CAD build for the part. Positions are in the model's coordinates, mm. Face numbers are marked on the shaded views. A direction names the side the tool comes from. Give positions to 0.01 mm unless a question says otherwise; leave off trailing zeros. Order: outer loops, then holes, each group sorted by start corner. A loop starts at its lowest first (then second) coordinate and runs counter-clockwise, first axis right, second up. Notation, with made-up numbers: (18, 16) -> (24, 16) arc R24 ccw to (24, 50) -> close; hole circle Ø1 at (17.5, 10.5). An arc over 180 degrees is marked (long way). Use one line per item in the form item = value. Start each with the question number.
1) Drop flat-ended pins along their axis: P1, Ø10, axis at y = 17.5, z = 31, coming from the +X side; P2, Ø3.5, axis at x = -60, y = 37, coming from the +Z side; P3, Ø0.9, axis at x = 60.5, y = -37, coming from the +Z side; P4, Ø1, axis at x = 59, z = 25.5, coming from the -Y side. Give the stop position or say it passes through.
2) Cut at A-A, the plane y = 0. State how many separate pieces and enclosed holes the cut face has, and give its area (3 significant figures).
3) Cut at B-B, the plane z = 23. Give the cut face in (x, y), and give its area (3 significant figures).
4) Mould opens along Y. For the marked faces 1, 2 and 3 say: pulls with the +Y half, pulls with the -Y half, needs draft (parallel to the pull), parting line crosses it, or undercut.
5) Tool access for the marked faces 4, 5, 6 and 7: list every direction of +Z, -Z, +X, -X, +Y, -Y with a clear straight run to the whole face (end or side of a thin tool).
6) Probe line 1 (Y direction, x = 60, z = 23); line 2 (Y direction, x = 45, z = 26); line 3 (X direction, y = 7.5, z = 14.5). List the from-to ranges inside material, lowest first.
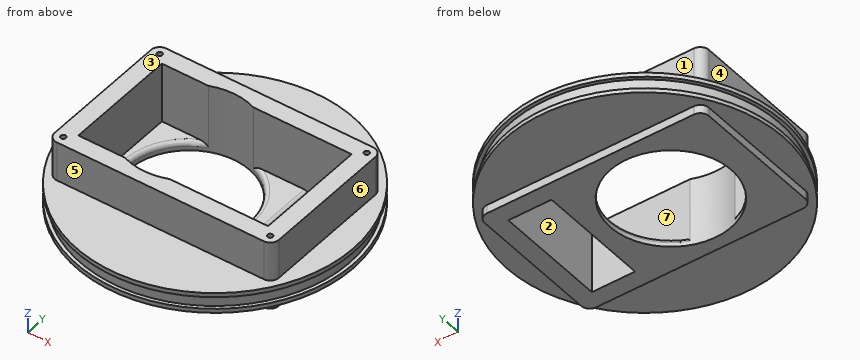
from build123d import *

# Parameters (mm, degrees)
SKETCH1_W           = 130
SKETCH1_H           = 85
SKETCH1_W_2         = 110
SKETCH1_H_2         = 65
BOSS_EXTRUDE1_DEPTH = 35
SKETCH2_W           = 130
SKETCH2_H           = 85
SKETCH2_R           = 35
SKETCH2_W_2         = 25
SKETCH2_H_2         = 65
BOSS_EXTRUDE2_DEPTH = 5
CUT_EXTRUDE1_START  = 45
SKETCH2_2_R         = 35
CUT_EXTRUDE1_DEPTH  = 45
SKETCH3_R           = 1.5
CUT_EXTRUDE2_DEPTH  = 15
FILLET1_R           = 5
FILLET2_R           = 2.5
SKETCH4_R           = 80
BOSS_EXTRUDE3_DEPTH = 12
SKETCH5_W           = 7
SKETCH5_H           = 2


with BuildPart() as part:
    # Sketch1 → Boss-Extrude1 (new body)
    with BuildSketch(Plane.XY):
        Rectangle(SKETCH1_W, SKETCH1_H)
        Rectangle(SKETCH1_W_2, SKETCH1_H_2, mode=Mode.SUBTRACT)
    extrude(amount=BOSS_EXTRUDE1_DEPTH)

    # Sketch2 → Boss-Extrude2 (add)
    with BuildSketch(Plane.XY):
        Rectangle(SKETCH2_W, SKETCH2_H)
        with Locations((-15, 0)):
            Circle(SKETCH2_R, mode=Mode.SUBTRACT)
        with Locations((42.5, 0)):
            Rectangle(SKETCH2_W_2, SKETCH2_H_2, mode=Mode.SUBTRACT)
    extrude(amount=-BOSS_EXTRUDE2_DEPTH)

    # Sketch2_2 → Cut-Extrude1 (cut)
    with BuildSketch(Plane.XY.offset(CUT_EXTRUDE1_START)):
        with Locations((-15, 0)):
            Circle(SKETCH2_2_R)
    extrude(amount=-CUT_EXTRUDE1_DEPTH, mode=Mode.SUBTRACT)

    # Sketch3 → Cut-Extrude2 (cut)
    with BuildSketch(Plane.XY.offset(35)):
        with Locations((-60, 37.5)):
            Circle(SKETCH3_R)
        with Locations((60, 37.5)):
            Circle(SKETCH3_R)
        with Locations((-60, -37.5)):
            Circle(SKETCH3_R)
        with Locations((60, -37.5)):
            Circle(SKETCH3_R)
    extrude(amount=-CUT_EXTRUDE2_DEPTH, mode=Mode.SUBTRACT)

    # Fillet1
    fillet1_edges = [part.edges().sort_by_distance(p)[0] for p in [
        (65, -42.5, 15),
        (-65, -42.5, 15),
        (-65, 42.5, 15),
        (65, 42.5, 15),
    ]]
    fillet(fillet1_edges, radius=FILLET1_R)

    # Fillet2
    fillet2_edges = [part.edges().sort_by_distance(p)[0] for p in [
        (-50, 0, 0),
        (13.979849352, 19.625705886, 0),
        (30, 0, 0),
    ]]
    fillet(fillet2_edges, radius=FILLET2_R)

    # Sketch4 → Boss-Extrude3 (add)
    with BuildSketch(Plane.XY):
        Circle(SKETCH4_R)
        Polygon((60, 42.5), (-60, 42.5), (-65, 37.5), (-65, -37.5), (-60, -42.5), (60, -42.5), (65, -37.5), (65, 37.5), align=None, mode=Mode.SUBTRACT)
    extrude(amount=BOSS_EXTRUDE3_DEPTH)

    # Sketch5 → Cut-Revolve1 (revolve, cut)
    with BuildSketch(Plane(origin=(0, 0, 0), x_dir=(0, 0, -1), z_dir=(1, 0, 0)), mode=Mode.PRIVATE) as cut_revolve1_sk:
        with Locations((-6, 79)):
            Rectangle(SKETCH5_W, SKETCH5_H)
    revolve(cut_revolve1_sk.sketch.rotate(Axis((0, 0, 0), (0, 0, -1)), 90), axis=Axis((0, 0, 0), (0, 0, -1)), mode=Mode.SUBTRACT)


solid = part.part
Result:
q1.P1 = 65
q1.P2 = 35
q1.P3 = 20
q1.P4 = -42.5
q2.separate_pieces = 3
q2.enclosed_holes = 0
q2.area = 1,200 mm²
q3.outline = (-65, -37.5) arc R5 ccw to (-60, -42.5) -> (60, -42.5) arc R5 ccw to (65, -37.5) -> (65, 37.5) arc R5 ccw to (60, 42.5) -> (-60, 42.5) arc R5 ccw to (-65, 37.5) -> close; hole circle Ø3 at (-60, -37.5); hole circle Ø3 at (-60, 37.5); hole (-55, -32.5) -> (-27.99, -32.5) arc R35 ccw to (-2.01, -32.5) -> (55, -32.5) -> (55, 32.5) -> (-2.01, 32.5) arc R35 ccw to (-27.99, 32.5) -> (-55, 32.5) -> close; hole circle Ø3 at (60, -37.5); hole circle Ø3 at (60, 37.5)
q3.area = 3,760 mm²
q4.face_1 = pulls with the +Y half
q4.face_2 = undercut
q4.face_3 = needs draft
q5.face_4 = +Z, -X, +Y, -Y
q5.face_5 = +Z, +X, -X, -Y
q5.face_6 = +Z, +X, +Y, -Y
q5.face_7 = +Z
q6.line_1 = -42.5 to -39, -36 to 36, 39 to 42.5
q6.line_2 = -42.5 to -32.5, 32.5 to 42.5
q6.line_3 = -65 to -55, 55 to 65
